from build123d import *

# Parameters (mm, degrees)
SKETCH_1_W           = 174.66
SKETCH_1_H           = 128.33
EXTRUDE_1_DEPTH      = 20
CUT_EXTRUDE_2_DEPTH  = 8
CUT_EXTRUDE_3_DEPTH  = 10.5
SKETCH_6_W           = 5.6
SKETCH_6_H           = 15.1
SKETCH_6_W_2         = 2.75
SKETCH_6_H_2         = 7.6
CUT_EXTRUDE_4_DEPTH  = 8
SKETCH_7_W           = 9.5
SKETCH_7_H           = 19.5
CUT_EXTRUDE_5_DEPTH  = 2
SKETCH_8_R           = 1.375
CUT_EXTRUDE_6_DEPTH  = 195.468071014
SKETCH_9_W           = 143.3
SKETCH_9_H           = 5.5
SKETCH_9_W_2         = 144.4
SKETCH_9_H_2         = 6.339108063
CUT_EXTRUDE_7_DEPTH  = 18
SKETCH_2_W           = 156.66
SKETCH_2_H           = 88.33
CUT_EXTRUDE_8_DEPTH  = 124.6337279
SKETCH_10_W          = 165
SKETCH_10_H          = 100
CUT_EXTRUDE_10_DEPTH = 7.5
SKETCH_11_W          = 44.991562028
SKETCH_11_H          = 7.165
CUT_EXTRUDE_11_DEPTH = 18
SKETCH_12_W          = 166
SKETCH_12_H          = 124.6
CUT_EXTRUDE_12_DEPTH = 13
SKETCH_13_W          = 150
SKETCH_13_H          = 124.6
CUT_EXTRUDE_15_DEPTH = 5
SKETCH_14_W          = 8
SKETCH_14_H          = 101
CUT_EXTRUDE_16_DEPTH = 5
SKETCH_15_W          = 3.06
SKETCH_15_H          = 128.33
SKETCH_15_W_2        = 1.6
CUT_EXTRUDE_17_DEPTH = 124.6337279
SKETCH_16_W          = 8
SKETCH_16_H          = 11.6
SKETCH_16_H_2        = 10.625891937
EXTRUDE_2_DEPTH      = 3.2


with BuildPart() as part:
    # 草图1 → 凸台-拉伸1 (new body)
    with BuildSketch(Plane.XY):
        with Locations((1.964925, -18.971725)):
            Rectangle(SKETCH_1_W, SKETCH_1_H)
    extrude(amount=EXTRUDE_1_DEPTH)

    # 草图4 → 切除-拉伸2 (cut)
    with BuildSketch(Plane(origin=(0, 0, 0), x_dir=(-1, 0, 0), z_dir=(0, 0, -1))):
        Polygon((-85.794925, 29.193275), (78.715075, 29.193275), (78.715075, -71.136725), (-16.794925, -71.136725), (-16.794925, -74.136725), (-61.794925, -74.136725), (-61.794925, -71.136725), (-85.794925, -71.136725), align=None)
    extrude(amount=-CUT_EXTRUDE_2_DEPTH, mode=Mode.SUBTRACT)

    # 草图5 → 切除-拉伸3 (cut)
    with BuildSketch(Plane(origin=(0, 0, 0), x_dir=(-1, 0, 0), z_dir=(0, 0, -1))):
        Polygon((-76.894925, 34.854166937), (71.505075, 34.854166937), (71.505075, 43.654166937), (80.305075, 43.654166937), (80.305075, 34.854166937), (80.305075, -72.145833063), (80.305075, -80.945833063), (69.505075, -80.945833063), (69.505075, -72.145833063), (-77.794925, -72.145833063), (-77.794925, -80.945833063), (-85.694925, -80.945833063), (-85.694925, -72.145833063), (-85.694925, 34.854166937), (-85.694925, 43.654166937), (-76.894925, 43.654166937), align=None)
    extrude(amount=-CUT_EXTRUDE_3_DEPTH, mode=Mode.SUBTRACT)

    # 草图6 → 切除-拉伸4 (cut)
    with BuildSketch(Plane(origin=(89.294925, 0, 0), x_dir=(0, 0, -1), z_dir=(1, 0, 0))):
        with Locations((-5.2, 23.104166937)):
            Rectangle(SKETCH_6_W, SKETCH_6_H)
        with Locations((-6.625, 4.954166937)):
            Rectangle(SKETCH_6_W_2, SKETCH_6_H_2)
        with Locations((-6.625, -6.145833063)):
            Rectangle(SKETCH_6_W_2, SKETCH_6_H_2)
    extrude(amount=-CUT_EXTRUDE_4_DEPTH, mode=Mode.SUBTRACT)

    # 草图7 → 切除-拉伸5 (cut)
    with BuildSketch(Plane(origin=(89.294925, 0, 0), x_dir=(0, 0, -1), z_dir=(1, 0, 0))):
        with Locations((-5.189589766, 23.17874546)):
            Rectangle(SKETCH_7_W, SKETCH_7_H)
    extrude(amount=-CUT_EXTRUDE_5_DEPTH, mode=Mode.SUBTRACT)

    # 草图8 → 切除-拉伸6 (cut, through all)
    with BuildSketch(Plane(origin=(89.294925, 0, 0), x_dir=(0, 0, -1), z_dir=(1, 0, 0))):
        with Locations(Location((-6.755495721, -13.945833063, 0), (0, 0, 90))):
            Circle(SKETCH_8_R)
        with Locations(Location((-6.755495721, -18.945833063, 0), (0, 0, 90))):
            Circle(SKETCH_8_R)
        with Locations(Location((-6.755495721, -23.945833063, 0), (0, 0, 90))):
            Circle(SKETCH_8_R)
        with Locations(Location((-6.755495721, -28.945833063, 0), (0, 0, 90))):
            Circle(SKETCH_8_R)
        with Locations(Location((-6.755495721, -33.945833063, 0), (0, 0, 90))):
            Circle(SKETCH_8_R)
        with Locations(Location((-6.755495721, -38.945833063, 0), (0, 0, 90))):
            Circle(SKETCH_8_R)
        with Locations(Location((-6.755495721, -43.945833063, 0), (0, 0, 90))):
            Circle(SKETCH_8_R)
        with Locations(Location((-6.755495721, -48.945833063, 0), (0, 0, 90))):
            Circle(SKETCH_8_R)
        with Locations(Location((-6.755495721, -53.945833063, 0), (0, 0, 90))):
            Circle(SKETCH_8_R)
        with Locations(Location((-6.755495721, -58.945833063, 0), (0, 0, 90))):
            Circle(SKETCH_8_R)
        with Locations(Location((-6.755495721, -63.945833063, 0), (0, 0, 90))):
            Circle(SKETCH_8_R)
        with Locations(Location((-6.755495721, -68.945833063, 0), (0, 0, 90))):
            Circle(SKETCH_8_R)
    extrude(amount=-CUT_EXTRUDE_6_DEPTH, mode=Mode.SUBTRACT)

    # 草图9 → 切除-拉伸7 (cut)
    with BuildSketch(Plane(origin=(0, 0, 0), x_dir=(-1, 0, 0), z_dir=(0, 0, -1))):
        with Locations((-4.144925, -78.386725)):
            Rectangle(SKETCH_9_W, SKETCH_9_H)
        with Locations((-2.694925, 40.023720969)):
            Rectangle(SKETCH_9_W_2, SKETCH_9_H_2)
    extrude(amount=-CUT_EXTRUDE_7_DEPTH, mode=Mode.SUBTRACT)

    # 草图2 → 切除-拉伸8 (cut, through all)
    with BuildSketch(Plane.XY.offset(20)):
        with Locations((0.964925, -16.971725)):
            Rectangle(SKETCH_2_W, SKETCH_2_H)
    extrude(amount=-CUT_EXTRUDE_8_DEPTH, mode=Mode.SUBTRACT)

    # 草图10 → 切除-拉伸10 (cut)
    with BuildSketch(Plane(origin=(0, 0, 10.5), x_dir=(-1, 0, 0), z_dir=(0, 0, -1))):
        with Locations((-0.964925, -16.971725)):
            Rectangle(SKETCH_10_W, SKETCH_10_H)
    extrude(amount=-CUT_EXTRUDE_10_DEPTH, mode=Mode.SUBTRACT)

    # 草图11 → 切除-拉伸11 (cut)
    with BuildSketch(Plane(origin=(0, 0, 0), x_dir=(-1, 0, 0), z_dir=(0, 0, -1))):
        with Locations((-39.290706014, -70.554225)):
            Rectangle(SKETCH_11_W, SKETCH_11_H)
    extrude(amount=-CUT_EXTRUDE_11_DEPTH, mode=Mode.SUBTRACT)

    # 草图12 → 切除-拉伸12 (cut)
    with BuildSketch(Plane(origin=(0, 0, 0), x_dir=(-1, 0, 0), z_dir=(0, 0, -1))):
        with Locations((-2.694925, -18.645833063)):
            Rectangle(SKETCH_12_W, SKETCH_12_H)
    extrude(amount=-CUT_EXTRUDE_12_DEPTH, mode=Mode.SUBTRACT)

    # 草图13 → 切除-拉伸15 (cut)
    with BuildSketch(Plane(origin=(0, 0, 13), x_dir=(-1, 0, 0), z_dir=(0, 0, -1))):
        with Locations((-2.694925, -18.645833063)):
            Rectangle(SKETCH_13_W, SKETCH_13_H)
    extrude(amount=-CUT_EXTRUDE_15_DEPTH, mode=Mode.SUBTRACT)

    # 草图14 → 切除-拉伸16 (cut)
    with BuildSketch(Plane(origin=(0, 0, 13), x_dir=(-1, 0, 0), z_dir=(0, 0, -1))):
        with Locations((76.305075, -18.845833063)):
            Rectangle(SKETCH_14_W, SKETCH_14_H)
        with Locations((-81.694925, -18.845833063)):
            Rectangle(SKETCH_14_W, SKETCH_14_H)
    extrude(amount=-CUT_EXTRUDE_16_DEPTH, mode=Mode.SUBTRACT)

    # 草图15 → 切除-拉伸17 (cut, through all)
    with BuildSketch(Plane(origin=(0, 0, 0), x_dir=(-1, 0, 0), z_dir=(0, 0, -1))):
        with Locations((83.835075, -18.971725)):
            Rectangle(SKETCH_15_W, SKETCH_15_H)
        with Locations((-88.494925, -18.971725)):
            Rectangle(SKETCH_15_W_2, SKETCH_15_H)
    extrude(amount=-CUT_EXTRUDE_17_DEPTH, mode=Mode.SUBTRACT)

    # 草图16 → 凸台-拉伸2 (add)
    with BuildSketch(Plane(origin=(0, 0, 13), x_dir=(-1, 0, 0), z_dir=(0, 0, -1))):
        with Locations((76.305075, -75.145833063)):
            Rectangle(SKETCH_16_W, SKETCH_16_H)
        with Locations((-81.694925, -75.145833063)):
            Rectangle(SKETCH_16_W, SKETCH_16_H)
        with Locations((76.305075, 38.341220968)):
            Rectangle(SKETCH_16_W, SKETCH_16_H_2)
        with Locations((-81.694925, 38.341220968)):
            Rectangle(SKETCH_16_W, SKETCH_16_H_2)
    extrude(amount=EXTRUDE_2_DEPTH)


solid = part.part
For this review, take the finished solid that the model builds, in its own axes (mm). A direction names the side the tool comes from. Round coordinates to 2 decimals unless told otherwise and drop trailing zeros. Loops run counter-clockwise (first coordinate to the right, second up) from the corner with the lowest first, then second, coordinate; pieces in that order, holes last. Notation, with made-up numbers: (-3.5, 82.5) - (16.5, 82.5) arc R13 cw to (16.5, 90.5) - close; hole circle Ø4 at (-34.75, 1.5). An arc over 180 degrees is marked (long way). One line per question, with ' | ' between items.
Q1. Take a section at A-A (x = 52.5). Give the boundary of the cut face in (y, z), and give its area (3 significant figures).
Taken from the geometry:
outline: (-83.14, 0) - (-81.14, 0) - (-81.14, 18) - (-61.14, 18) - (-61.14, 20) - (-83.14, 20) - close; (27.19, 18) - (43.65, 18) - (43.65, 0) - (45.19, 0) - (45.19, 20) - (27.19, 20) - close | area: 144 mm²
Q2. For line 1 along X through (y, z) = (-36.5, 9.25); line 2 along Y through (x, z) = (-69.5, 7); line 3 along X through (y, z) = (14.5, 11.5), list the stretches that pass through material, from the lowest coordinate up. Write a range as [from, to].
Taken from the geometry:
line 1: x = [-82.31, -80.31], [85.69, 87.69] | line 2: y = [-83.14, -80.95], [43.65, 45.19] | line 3: x = [-82.31, -81.54], [85.69, 87.69]
Q3. For pin 1 (1.6 mm diameter, centred on y = -63.95, z = 6.76, fed in from -X) (3 decimals); pin 2 (6.5 mm diameter, centred on x = 82, y = 36, fed in from -Z), all flat-tipped, find the tip position at first contact; note any pin that passes through.
Taken from the geometry:
pin 1: passes through | pin 2: stops at z = 9.8
Q4. Tool access review of faces 4 (the flat face through (87.295, 23, 2)), 5 (the flat face through (-81.535, -18, 14)), 6 (the flat face through (82, -69.346, 14)), 7 (the flat face through (2, -83.137, 10)): name each direction out of +Z, -Z, +X, -X, +Y, -Y from which nothing blocks a thin tool from reaching the whole face with its end or side.
Taken from the geometry:
face 4: +X | face 5: none | face 6: -Z | face 7: +Z, -Z, +X, -X, -Y
Q5. The part is to be moulded in two halves that separate along X. For faces 1 (the flat face through (-10.3, -61.4, 20)), 2 (the flat face through (-82.305, -20, 10)), 3 (the flat face through (-80.305, -20, 5)), say which applies: released by +X, released by -X, zero draft, split by the parting line, or undercut.
Taken from the geometry:
face 1: zero draft | face 2: released by -X | face 3: undercut
